Read the model definition and answer for the solid it produces. Units are mm, in the model's axes. Face numbers are marked on the shaded views. A direction names the side the tool comes from. Round coordinates to 2 decimals unless told otherwise and drop trailing zeros. Write each loop counter-clockwise with the first axis right and the second up, starting at its lowest first coordinate (ties: lowest second). Pieces come first, ordered by that corner, then holes.
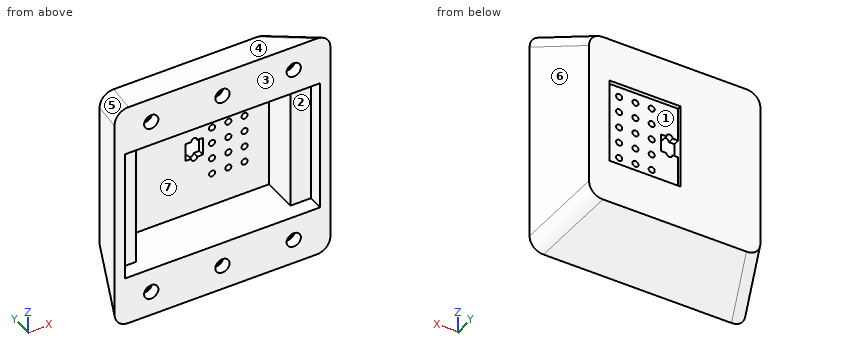
from build123d import *

# Parameters (mm, degrees)
TOP_ENCLOSURE_DEPTH                     = 65
TOP_EXTRA_DEPTH                         = 10
SKETCH3_W                               = 35
SKETCH3_H                               = 42
SOLAR_CELL_SLOT_DEPTH                   = 2
SKETCH4_R                               = 1.5
SOLAR_CELL_HOLES_DEPTH                  = 97.010416102
BOSS_EXTRUDE1_REACH                     = 97.584
BOSS_EXTRUDE2_REACH                     = 108.913
FILLET1_R                               = 7.5
CBORE_FOR_M5_HEX_HEAD_BOLT1_D           = 5.3
CBORE_FOR_M5_HEX_HEAD_BOLT1_DEPTH       = 10
CBORE_FOR_M5_HEX_HEAD_BOLT1_CBORE_D     = 7
CBORE_FOR_M5_HEX_HEAD_BOLT1_CBORE_DEPTH = 5


with BuildPart() as part:
    # Master_Geometry → Top_Enclosure (new body)
    with BuildSketch(Plane.XY):
        Polygon((-48, -3.5), (-53, -3.5), (-42.080892972, 26.5), (42.080892972, 26.5), (53, -3.5), (48, -3.5), (48, 4), (38, 4), (38, 21.5), (-38, 21.5), (-38, 4), (-48, 4), align=None)
    extrude(amount=TOP_ENCLOSURE_DEPTH)

    # Sketch2 → Top_Extra (add)
    with BuildSketch(Plane.XY.offset(65)):
        Polygon((-42.080892972, 26.5), (42.080892972, 26.5), (53, -3.5), (-53, -3.5), align=None)
    top_extra = extrude(amount=TOP_EXTRA_DEPTH)

    # Mirror1: Top_Extra across plane
    add(top_extra.mirror(Plane(origin=(0, 0, 32.5), x_dir=(1, 0, 0), z_dir=(0, 0, -1))))

    # Sketch3 → Solar_Cell_Slot (cut)
    with BuildSketch(Plane(origin=(0, 26.5, 0), x_dir=(1, 0, 0), z_dir=(0, 1, 0))):
        with Locations((14.580892972, -32.5)):
            Rectangle(SKETCH3_W, SKETCH3_H)
    extrude(amount=-SOLAR_CELL_SLOT_DEPTH, mode=Mode.SUBTRACT)

    # Sketch4 → Solar_Cell_Holes (cut, through all)
    with BuildSketch(Plane(origin=(0, 24.5, 0), x_dir=(1, 0, 0), z_dir=(0, 1, 0))):
        with Locations(Location((10.080892972, -32.5, 0), (0, 0, 270))):
            Circle(SKETCH4_R)
        with Locations(Location((18.080892972, -32.5, 0), (0, 0, 270))):
            Circle(SKETCH4_R)
        with Locations(Location((26.080892972, -32.5, 0), (0, 0, 270))):
            Circle(SKETCH4_R)
        with Locations(Location((10.080892972, -40.5, 0), (0, 0, 270))):
            Circle(SKETCH4_R)
        with Locations(Location((18.080892972, -40.5, 0), (0, 0, 270))):
            Circle(SKETCH4_R)
        with Locations(Location((26.080892972, -40.5, 0), (0, 0, 270))):
            Circle(SKETCH4_R)
        with Locations(Location((10.080892972, -48.5, 0), (0, 0, 270))):
            Circle(SKETCH4_R)
        with Locations(Location((18.080892972, -48.5, 0), (0, 0, 270))):
            Circle(SKETCH4_R)
        with Locations(Location((26.080892972, -48.5, 0), (0, 0, 270))):
            Circle(SKETCH4_R)
        with Locations(Location((10.080892972, -24.5, 0), (0, 0, 270))):
            Circle(SKETCH4_R)
        with Locations(Location((18.080892972, -24.5, 0), (0, 0, 270))):
            Circle(SKETCH4_R)
        with Locations(Location((26.080892972, -24.5, 0), (0, 0, 270))):
            Circle(SKETCH4_R)
        with Locations(Location((10.080892972, -16.5, 0), (0, 0, 270))):
            Circle(SKETCH4_R)
        with Locations(Location((18.080892972, -16.5, 0), (0, 0, 270))):
            Circle(SKETCH4_R)
        with Locations(Location((26.080892972, -16.5, 0), (0, 0, 270))):
            Circle(SKETCH4_R)
        with BuildLine():
            Line((2.830892972, -28.125), (5.580892972, -28.125))
            Line((5.580892972, -28.125), (5.580892972, -36.875))
            Line((5.580892972, -36.875), (2.830892972, -36.875))
            ThreePointArc((2.830892972, -36.875), (1.330892972, -38.375), (-0.169107028, -36.875))
            Line((-0.169107028, -36.875), (-2.919107028, -36.875))
            Line((-2.919107028, -36.875), (-2.919107028, -28.125))
            Line((-2.919107028, -28.125), (-0.169107028, -28.125))
            ThreePointArc((-0.169107028, -28.125), (1.330892972, -26.625), (2.830892972, -28.125))
        make_face()
    extrude(amount=-SOLAR_CELL_HOLES_DEPTH, mode=Mode.SUBTRACT)

    # Boss-Extrude1: up to this plane
    boss_extrude1_end = Plane(origin=(42.080892972, 26.5, 65), z_dir=(-0.9396926207859069, -0.3420201433256729, 0))
    # Sketch5 → Boss-Extrude1 (add, up to the surface)
    with BuildSketch(Plane(origin=(0, 0, 0), x_dir=(0, 0, -1), z_dir=(1, 0, 0)), mode=Mode.PRIVATE) as boss_extrude1_sk1:
        Polygon((-75, 26.5), (-75, -3.5), (-88.989229745, -3.5), align=None)
    boss_extrude1_tool1 = split(extrude(boss_extrude1_sk1.sketch, amount=BOSS_EXTRUDE1_REACH, mode=Mode.PRIVATE), bisect_by=boss_extrude1_end, keep=Keep.BOTH, mode=Mode.PRIVATE)
    boss_extrude1 = boss_extrude1_tool1.solids().sort_by_distance((0, 6.5, 79.663077))[0]
    add(boss_extrude1)

    # Boss-Extrude2: up to this face of the body (flat: up to its plane)
    boss_extrude2_end = Plane(part.part.faces().sort_by_distance((-47.540446486, 11.5, 32.5))[0])
    # Sketch6 → Boss-Extrude2 (add, up to the picked face)
    with BuildSketch(Plane.ZY, mode=Mode.PRIVATE) as boss_extrude2_sk1:
        Polygon((75, 26.5), (88.989229745, -3.5), (75, -3.5), align=None)
    boss_extrude2_tool1 = split(extrude(boss_extrude2_sk1.sketch, amount=BOSS_EXTRUDE2_REACH, mode=Mode.PRIVATE), bisect_by=boss_extrude2_end, keep=Keep.BOTH, mode=Mode.PRIVATE)
    boss_extrude2 = boss_extrude2_tool1.solids().sort_by(Axis((0, 6.5, 79.663077), (-1, 0, 0)))[0]
    add(boss_extrude2)

    # Mirror3: Boss-Extrude1, Boss-Extrude2 across plane
    add(boss_extrude1.mirror(Plane(origin=(0, 0, 32.5), x_dir=(1, 0, 0), z_dir=(0, 0, -1))))
    add(boss_extrude2.mirror(Plane(origin=(0, 0, 32.5), x_dir=(1, 0, 0), z_dir=(0, 0, -1))))

    # Fillet1
    fillet1_edges = [part.edges().sort_by_distance(p)[0] for p in [
        (47.540446486, 11.5, 81.994614872),
        (-47.540446486, 11.5, 81.994614872),
        (47.540446486, 11.5, -16.994614872),
        (-47.540446486, 11.5, -16.994614872),
    ]]
    fillet(fillet1_edges, radius=FILLET1_R)

    # CBORE for M5 Hex Head Bolt1
    with Locations(Plane(origin=(0, -3.5, 0), x_dir=(-1, 0, 0), z_dir=(0, -1, 0))):
        with Locations((35, -76.989229745), (0, -76.989229745), (-35, -76.989229745), (-35, 11.989229745), (0, 11.989229745), (35, 11.989229745)):
            CounterBoreHole(CBORE_FOR_M5_HEX_HEAD_BOLT1_D / 2, CBORE_FOR_M5_HEX_HEAD_BOLT1_CBORE_D / 2, CBORE_FOR_M5_HEX_HEAD_BOLT1_CBORE_DEPTH, depth=CBORE_FOR_M5_HEX_HEAD_BOLT1_DEPTH)


solid = part.part
Q1. Which of the six approach directions +Z, -Z, +X, -X, +Y, -Y give full straight-line access (tool end or side, diameter ignored) to the marked faces 1, 2 and 3?
Verdict:
face 1: +Y
face 2: -Y
face 3: +Z, -Z, +X, -X, -Y
Q2. Section B-B (x = -16.5) is taken. Determine the outline of the cut face in (y, z).
Verdict:
outline: (-3.5, -23.99) - (26.5, -10) - (26.5, 75) - (-3.5, 88.99) - (-3.5, 65) - (21.5, 65) - (21.5, 0) - (-3.5, 0) - close
Q3. Section D-D (z = 61) is taken. Determine the outline of the cut face in (x, y), then the cut area to 3 significant figures.
Verdict:
outline: (-53, -3.5) - (-48, -3.5) - (-48, 4) - (-38, 4) - (-38, 21.5) - (38, 21.5) - (38, 4) - (48, 4) - (48, -3.5) - (53, -3.5) - (42.08, 26.5) - (-42.08, 26.5) - close
area: 802 mm2
Q4. Section A-A (z = 32.5) is taken. State how many separate pieces and enclosed holes the cut face has, then the cut area to 3 significant figures.
Verdict:
separate pieces: 5
enclosed holes: 0
area: 680 mm2
Q5. Section C-C (z = 16.5) is taken. Determine the outline of the cut face in (x, y), then the cut area to 3 significant figures.
Verdict:
outline: (-53, -3.5) - (-48, -3.5) - (-48, 4) - (-38, 4) - (-38, 21.5) - (8.58, 21.5) - (8.58, 24.5) - (-2.92, 24.5) - (-2.92, 26.5) - (-42.08, 26.5) - close; (11.58, 21.5) - (16.58, 21.5) - (16.58, 24.5) - (11.58, 24.5) - close; (19.58, 21.5) - (24.58, 21.5) - (24.58, 24.5) - (19.58, 24.5) - close; (27.58, 21.5) - (38, 21.5) - (38, 4) - (48, 4) - (48, -3.5) - (53, -3.5) - (42.08, 26.5) - (32.08, 26.5) - (32.08, 24.5) - (27.58, 24.5) - close
area: 705 mm2
Q6. Flat-ended cylindrical pins translate along their axes: pin 1 Ø12 at (x, y) = (-13, 4.5) entering from -Z; pin 2 Ø8 at (x, z) = (-44.5, 26) entering from -Y; pin 3 Ø3 at (y, z) = (2, 24) entering from +X; pin 4 Ø1.5 at (y, z) = (17, 39.5) entering from +X. Find the tip coordinate at first contact, or state that the pin passes through.
Verdict:
pin 1: stops at z = -23.06
pin 2: stops at y = -3.5
pin 3: stops at x = 51.54
pin 4: stops at x = 45.81
Q7. Straight lines are drawn through the part: probe 1 along Z at (x, y) = (37, 4.5); probe 2 along Z at (x, y) = (35, 3.85); probe 3 along X at (y, z) = (23.55, 24.5). For each, find the intervals that lie inside material, in ascending order.
Verdict:
probe 1: z = -20.26 to -13.73, -10.25 to 0, 65 to 75.25, 78.73 to 85.26
probe 2: z = -20.56 to -14.64, -9.34 to 0, 65 to 74.34, 79.64 to 85.56
probe 3: x = -43.15 to 8.58, 11.58 to 16.58, 19.58 to 24.58, 27.58 to 43.15
Q8. Determine the mould class of the marked faces 4, 5, 6 and 7 for opening direction X: pulls with the +X half, pulls with the -X half, needs draft (parallel to the pull), parting line crosses it, or undercut.
Verdict:
face 4: needs draft
face 5: pulls with the -X half
face 6: pulls with the +X half
face 7: undercut
